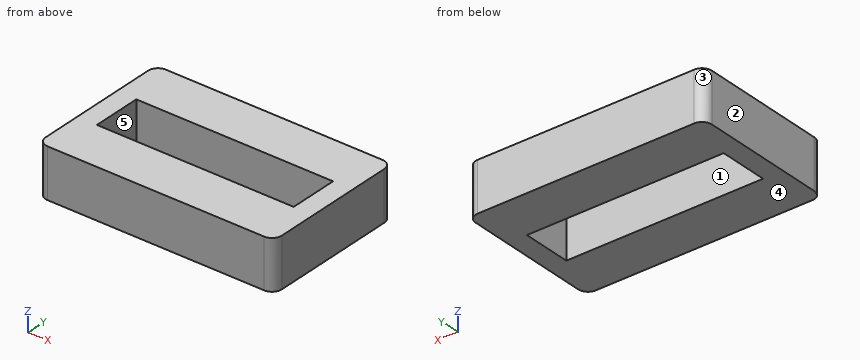
```python
from build123d import *

# Parameters (mm, degrees)
SKETCH1_W           = 24
SKETCH1_H           = 5
BOSS_EXTRUDE1_DEPTH = 15
SKETCH2_W           = 20
SKETCH2_H           = 5
CUT_EXTRUDE1_DEPTH  = 15
FILLET2_R           = 1


with BuildPart() as part:
    # Sketch1 → Boss-Extrude1 (new body)
    with BuildSketch(Plane(origin=(0, 0, 0), x_dir=(1, 0, 0), z_dir=(0, 1, 0))):
        Rectangle(SKETCH1_W, SKETCH1_H)
    extrude(amount=BOSS_EXTRUDE1_DEPTH)

    # Sketch2 → Cut-Extrude1 (cut)
    with BuildSketch(Plane(origin=(0, 0, -2.5), x_dir=(-1, 0, 0), z_dir=(0, 0, -1))):
        with Locations((0, 7.5)):
            Rectangle(SKETCH2_W, SKETCH2_H)
    extrude(amount=-CUT_EXTRUDE1_DEPTH, mode=Mode.SUBTRACT)

    # Fillet2
    fillet2_edges = [part.edges().sort_by_distance(p)[0] for p in [
        (12, 15, 0),
        (-12, 15, 0),
        (12, 0, 0),
        (-12, 0, 0),
    ]]
    fillet(fillet2_edges, radius=FILLET2_R)


solid = part.part
```
CAD build for the part. Positions are in the model's coordinates, mm. Face numbers are marked on the shaded views. A direction names the side the tool comes from. Round coordinates to 2 decimals unless told otherwise and drop trailing zeros. Order: outer loops, then holes, each group sorted by start corner. A loop starts at its lowest first (then second) coordinate and runs counter-clockwise, first axis right, second up. Notation, with made-up numbers: (0.5, -15.5) - (39.5, -15.5) arc R26 cw to (39.5, -1.5) - close; hole circle Ø4 at (-4.75, 35). An arc over 180 degrees is marked (long way). Use CSV: the item, a comma, the result in double quotes. Start each with the question number.
1) Tool access for the marked faces 1 and 2: list every direction of +Z, -Z, +X, -X, +Y, -Y with a clear straight run to the whole face (end or side of a thin tool).
2) Saw through at C-C (x = 5.25). List the corners of the cut face in (y, z).
3) Two-plate mould, pull along X, no slides. Class the marked faces 3, 4 and 5: pulls with the +X half, pulls with the -X half, needs draft (parallel to the pull), parting line crosses it, or undercut.
4) Wall check: L1, parallel to Y at x = 0.5, z = -1.6; L2, parallel to X at y = 9.5, z = -0.6. Give the ranges that are in metal, low to high. Write a range as [from, to].
5) Pin check, flat tip, straight feed: pin 1 Ø6 at (x, y) = (-2.5, 7.5) entering from -Z. Stop position of the tip, or through.
6) Saw through at A-A (y = 9). List the corners of the cut face in (x, z).
7) Saw through at B-B (z = 2). List the corners of the cut face in (x, y), and give its area (3 significant figures).
Values follow:
1,face 1,"+Z, -Z"
1,face 2,"+Z, -Z, -X, +Y, -Y"
2,outline,"(0, -2.5) - (5, -2.5) - (5, 2.5) - (0, 2.5) - close; (10, -2.5) - (15, -2.5) - (15, 2.5) - (10, 2.5) - close"
3,face 3,"pulls with the -X half"
3,face 4,"needs draft"
3,face 5,"undercut"
4,L1,"y = [0, 5], [10, 15]"
4,L2,"x = [-12, -10], [10, 12]"
5,pin 1,"stops at z = -2.5"
6,outline,"(-12, -2.5) - (-10, -2.5) - (-10, 2.5) - (-12, 2.5) - close; (10, -2.5) - (12, -2.5) - (12, 2.5) - (10, 2.5) - close"
7,outline,"(-12, 1) arc R1 ccw to (-11, 0) - (11, 0) arc R1 ccw to (12, 1) - (12, 14) arc R1 ccw to (11, 15) - (-11, 15) arc R1 ccw to (-12, 14) - close; hole (-10, 5) - (10, 5) - (10, 10) - (-10, 10) - close"
7,area,"259 mm2"
